```python
from build123d import *

# Parameters (mm, degrees)
SKETCH1_W           = 30
SKETCH1_H           = 10.5
BOSS_EXTRUDE1_DEPTH = 3
SKETCH2_W           = 30
SKETCH2_H           = 4
BOSS_EXTRUDE2_DEPTH = 37
SKETCH3_R           = 1.575
CUT_EXTRUDE1_DEPTH  = 41.268629229
SKETCH4_R           = 1.575
CUT_EXTRUDE2_DEPTH  = 41.268629229
FILLET1_R           = 5
SKETCH5_R           = 1.25
CUT_EXTRUDE3_DEPTH  = 44.991476447


with BuildPart() as part:
    # Sketch1 → Boss-Extrude1 (new body)
    with BuildSketch(Plane(origin=(0, 0, 0), x_dir=(1, 0, 0), z_dir=(0, 1, 0))):
        Rectangle(SKETCH1_W, SKETCH1_H)
    extrude(amount=BOSS_EXTRUDE1_DEPTH)

    # Sketch2 → Boss-Extrude2 (add)
    with BuildSketch(Plane(origin=(0, 3, 0), x_dir=(1, 0, 0), z_dir=(0, 1, 0))):
        with Locations((0, -3.25)):
            Rectangle(SKETCH2_W, SKETCH2_H)
    extrude(amount=BOSS_EXTRUDE2_DEPTH)

    # Sketch3 → Cut-Extrude1 (cut, through all)
    with BuildSketch(Plane(origin=(0, 3, 0), x_dir=(1, 0, 0), z_dir=(0, 1, 0))):
        with Locations(Location((-10.5, 2.05, 0), (0, 0, 270))):
            Circle(SKETCH3_R)
    extrude(amount=-CUT_EXTRUDE1_DEPTH, mode=Mode.SUBTRACT)

    # Sketch4 → Cut-Extrude2 (cut, through all)
    with BuildSketch(Plane(origin=(0, 3, 0), x_dir=(1, 0, 0), z_dir=(0, 1, 0))):
        with Locations(Location((10.5, 2.05, 0), (0, 0, 270))):
            Circle(SKETCH4_R)
    extrude(amount=-CUT_EXTRUDE2_DEPTH, mode=Mode.SUBTRACT)

    # Fillet1
    fillet1_edges = [part.edges().sort_by_distance(p)[0] for p in [
        (-15, 40, 3.25),
        (15, 40, 3.25),
    ]]
    fillet(fillet1_edges, radius=FILLET1_R)

    # Sketch5 → Cut-Extrude3 (cut, through all)
    with BuildSketch(Plane.XY.offset(5.25)):
        with Locations((0, 28.5)):
            Circle(SKETCH5_R)
    extrude(amount=-CUT_EXTRUDE3_DEPTH, mode=Mode.SUBTRACT)


solid = part.part
```
Read the model definition and answer for the solid it produces. Units are mm, in the model's axes. A direction names the side the tool comes from. Coordinates: 2 decimals unless noted, no trailing zeros. Order: outer loops, then holes, each group sorted by start corner. A loop starts at its lowest first (then second) coordinate and runs counter-clockwise, first axis right, second up. Notation, with made-up numbers: (27.25, 3) - (64.25, 3) arc R23 ccw to (64.25, 19) - close; hole circle Ø1 at (-32, 54.5). An arc over 180 degrees is marked (long way). Answer as a JSON object with one key per item and string values. Group by question number.
Item 1: Section B-B (z = -2.05) is taken. Give the vertices of the cut face in (x, y) (3 decimals).
Item 2: Section D-D (y = 21) is taken. Give the vertices of the cut face in (x, z), plus the area to 3 significant figures.
Item 3: Section A-A (y = 28.5) is taken. Give the vertices of the cut face in (x, z).
Item 4: A tool of negligible diameter and unlimited length cuts with its end or side. For faces 1 (the face through (0, 3, -2)), 2 (the face through (0, 0, 0)), from which of +Z, -Z, +X, -X, +Y, -Y can it reach the whole face along a straight path? Write none if from no direction.
Item 5: Consider probe 1 along X at (y, z) = (1.3, -2.05) (3 decimals); probe 2 along Y at (x, z) = (0, 3.65); probe 3 along Z at (x, y) = (-6, 14.5). Determine where each line is inside the solid, lowest interval first. Write a range as from..to.
Item 6: The mould has two halves that part along X. Classify faces 3 (the face through (-14, 38, 3)), 4 (the face through (0, 21, 1.25)), 5 (the face through (-0.27, 27.28, 3.28)), 6 (the face through (9.54, 1.52, -3.3)): +X half, -X half, draft (parallel to the pull), parting line (faces both ways), or undercut.
Item 7: Section C-C (x = 0) is taken. Give the vertices of the cut face in (y, z).
Item 8: Flat-ended cylindrical pins translate along their axes: P1, Ø4, axis at x = 2.5, y = 8, coming from the -Z side; P2, Ø3.5, axis at x = -10.5, z = -2.05, coming from the -Y side; P3, Ø2, axis at y = 32.5, z = -1.5, coming from the +X side; P4, Ø1, axis at x = -12, z = 0.5, coming from the +Y side. Find the tip coordinate at first contact, or state that the pin passes through.
Results are:
{
 "1": {"outline": "(-15, 0) - (-12.075, 0) - (-12.075, 3) - (-15, 3) - close; (-8.925, 0) - (8.925, 0) - (8.925, 3) - (-8.925, 3) - close; (12.075, 0) - (15, 0) - (15, 3) - (12.075, 3) - close"},
 "2": {"outline": "(-15, 1.25) - (15, 1.25) - (15, 5.25) - (-15, 5.25) - close", "area": "120 mm^2"},
 "3": {"outline": "(-15, 1.25) - (-1.25, 1.25) - (-1.25, 5.25) - (-15, 5.25) - close; (1.25, 1.25) - (15, 1.25) - (15, 5.25) - (1.25, 5.25) - close"},
 "4": {"face 1": "-Z, +X, -X, +Y", "face 2": "+Z, -Z, +X, -X, -Y"},
 "5": {"probe 1": "x = -15..-12.075, -8.925..8.925, 12.075..15", "probe 2": "y = 0..27.25, 29.75..40", "probe 3": "z = 1.25..5.25"},
 "6": {"face 3": "-X half", "face 4": "draft", "face 5": "undercut", "face 6": "undercut"},
 "7": {"outline": "(0, -5.25) - (3, -5.25) - (3, 1.25) - (27.25, 1.25) - (27.25, 5.25) - (0, 5.25) - close; (29.75, 1.25) - (40, 1.25) - (40, 5.25) - (29.75, 5.25) - close"},
 "8": {"P1": "stops at z = 1.25", "P2": "stops at y = 0", "P3": "passes through", "P4": "stops at y = 3"}
}
